Autodesk Inventor part; units mm, degrees
ref_plane "YZ Plane" through (0, 0, 0) normal (1, 0, 0) x (0, 1, 0)
ref_plane "XZ Plane" through (0, 0, 0) normal (0, 1, 0) x (-1, 0, 0)
ref_plane "XY Plane" through (0, 0, 0) normal (0, 0, 1) x (1, 0, 0)
sketch "スケッチ1" plane through (0, 0, 0) normal (0, 1, 0) x (-1, 0, 0)
  line L0 (7.8325, 11.4458) -> (-8.7675, 11.4458)
  line L1 (-8.7675, 11.4458) -> (-8.7675, -38.5542)
  line L2 (-8.7675, -38.5542) -> (7.8325, -38.5542)
  line L3 (7.8325, -38.5542) -> (7.8325, 11.4458)
  circle A0 centre (-0.4675, 6.9458) radius 2.5
  point P0 (0, 0)
  dimension "d0" = 16.6
  dimension "d1" = 5
  dimension "d2" = 8.3
  dimension "d3" = 8.3
  dimension "d4" = 4.5
  dimension "d5" = 2
  dimension "d6" = 50
extrude "押し出し1" add sketch "スケッチ1" along normal blind 3
sketch "スケッチ2" plane through (0, 3, 0) normal (0, 1, 0) x (1, 0, 0)
  line L0 (-7.8325, 38.5542) -> (-7.8325, -11.4458)
  line L1 (8.7675, -11.4458) -> (8.7675, 38.5542)
  line L2 (-7.8325, -11.4458) -> (8.7675, -11.4458)
  line L3 (8.7675, -11.4458) -> (8.7675, 38.5542)
  line L4 (8.7675, 38.5542) -> (-7.8325, 38.5542)
  line L5 (-7.8325, 38.5542) -> (-7.8325, -11.4458)
  circle A0 centre (0.4675, -6.9458) radius 1.5
  circle A1 centre (0.4675, -6.9458) radius 2.5
  point P0 (0, 0)
  dimension "d9" = 3
extrude "押し出し2" add sketch "スケッチ2" along normal blind 1 contours L4 L1 L2 L0 | A1
sketch "スケッチ3" plane through (0, 0, 0) normal (0, -1, 0) x (1, 0, 0)
  line L0 (-7.8325, -38.5542) -> (-7.8325, 11.4458)
  line L1 (8.7675, 11.4458) -> (8.7675, -38.5542)
  line L2 (-7.8325, -38.5542) -> (8.7675, -38.5542)
  line L3 (8.7675, -38.5542) -> (8.7675, -28.5542)
  line L4 (8.7675, -28.5542) -> (-7.8325, -28.5542)
  line L5 (-7.8325, -28.5542) -> (-7.8325, -38.5542)
  circle A0 centre (5.7675, -33.5542) radius 1.5
  circle A1 centre (-4.8325, -33.5542) radius 1.5
  point P0 (0, 0)
  dimension "d12" = 10
  dimension "d13" = 5
  dimension "d14" = 5
  dimension "d15" = 3
  dimension "d16" = 3
  dimension "d17" = 3
  dimension "d18" = 3
extrude "押し出し3" add sketch "スケッチ3" along normal blind 26.5
extrude "押し出し4" cut sketch "スケッチ3" against normal blind 21 contours A0 | A1
properties part number "armpart1"
The model under review builds one solid part; all positions refer to its coordinate system, in mm. A direction names the side the tool comes from. Coordinates: 2 decimals unless noted, no trailing zeros. Loops run counter-clockwise (first coordinate to the right, second up) from the corner with the lowest first, then second, coordinate; pieces in that order, holes last. Notation, with made-up numbers: (79.25, -28) -> (96.25, -28) arc R22 cw to (96.25, -15) -> close; hole circle Ø7 at (55, 40.5). An arc over 180 degrees is marked (long way). Answer as CSV lines item,"result".
Item 1: Take a section at C-C, the plane y = -3. State the section outline as (x, z) points, and give its area (3 significant figures).
Results below:
outline,"(-7.83, -38.55) -> (8.77, -38.55) -> (8.77, -28.55) -> (-7.83, -28.55) -> close; hole circle Ø3 at (-4.83, -33.55); hole circle Ø3 at (5.77, -33.55)"
area,"152 mm2"
Item 2: For L1, parallel to Z at x = 5.75, y = -7; L2, parallel to X at y = -6.5, z = -32.5; L3, parallel to Z at x = 1, y = -9.5, list the stretches that pass through material, from the lowest coordinate up.
Results below:
L1,"z = -38.55 to -35.05, -32.05 to -28.55"
L2,"x = -7.83 to -5.9, -3.77 to 4.7, 6.83 to 8.77"
L3,"z = -38.55 to -28.55"
Item 3: Draft analysis for pull direction Z (two halves, no side actions). For faces 1 (the cylindrical face through (0.793, 1.479, 4.467)), 2 (the flat face through (0, -11, -38.554)), 3 (the flat face through (1, 0, -8)), state which applies: +Z half, -Z half, draft (parallel to the pull), parting line (faces both ways), or undercut.
Results below:
face 1,"undercut"
face 2,"-Z half"
face 3,"draft"
Item 4: Take a section at B-B, the plane y = 1.5. State the section outline as (x, z) points, and give its area (3 significant figures).
Results below:
outline,"(-7.83, -38.55) -> (8.77, -38.55) -> (8.77, 11.45) -> (-7.83, 11.45) -> close; hole circle Ø3 at (-4.83, -33.55); hole circle Ø5 at (0.47, 6.95); hole circle Ø3 at (5.77, -33.55)"
area,"796 mm2"
Item 5: Insertion check: pin 1 (2.5 mm diameter, centred on x = 5.77, z = -33.55, fed in from -Y); pin 2 (4 mm diameter, centred on x = 0.47, z = 6.95, fed in from -Y); pin 3 (5.5 mm diameter, centred on x = 0.5, z = 7, fed in from -Y); pin 4 (5 mm diameter, centred on x = -2.5, y = -16, fed in from +Z). Each pin has a flat end and moves straight along its axis. Give the tip position at first contact, or say it passes through.
Results below:
pin 1,"passes through"
pin 2,"stops at y = 3"
pin 3,"stops at y = 0"
pin 4,"stops at z = -28.55"
Item 6: Machinability: for faces 4 (the flat face through (1, -13, -28.554)), 5 (the flat face through (2, 3, 8)), 6 (the cylindrical face through (0.272, 3.493, 8.433)), which of the approach directions +Z, -Z, +X, -X, +Y, -Y give a long, thin tool a straight path to every point of the face, cutting with its end or side? Answer none if there is none.
Results below:
face 4,"+Z, +X, -X, -Y"
face 5,"-Y"
face 6,"+Y, -Y"
Item 7: Take a section at A-A, the plane x = 6.25. State the section outline as (y, z) points.
Results below:
outline,"(-26.5, -38.55) -> (4, -38.55) -> (4, -34.97) -> (-26.5, -34.97) -> close; (-26.5, -32.13) -> (4, -32.13) -> (4, 11.45) -> (0, 11.45) -> (0, -28.55) -> (-26.5, -28.55) -> close"
Item 8: Take a section at D-D, the plane x = 0. State the section outline as (y, z) points, and give its area (3 significant figures).
Results below:
outline,"(-26.5, -38.55) -> (4, -38.55) -> (4, 5.52) -> (3, 5.52) -> (3, 4.49) -> (0, 4.49) -> (0, -28.55) -> (-26.5, -28.55) -> close; (0, 9.4) -> (3, 9.4) -> (3, 8.37) -> (4, 8.37) -> (4, 11.45) -> (0, 11.45) -> close"
area,"447 mm2"
